```python
from build123d import *

# Parameters (mm, degrees)
SKETCH2_R          = 30
CUT_EXTRUDE1_DEPTH = 40


with BuildPart() as part:
    # Sketch1 → Revolve1 (revolve)
    with BuildSketch(Plane.XY, mode=Mode.PRIVATE) as revolve1_sk:
        Polygon((0, 0), (0, 10), (-20, 10), (-20, 20), (-40, 20), (-40, 30), (-60, 30), (-60, 40), (-80, 40), (-80, 50), (-100, 50), (-100, 60), (-120, 60), (-120, 70), (-140, 70), (-140, 40), (-180, 40), (-180, 0), align=None)
    revolve(revolve1_sk.sketch.rotate(Axis((0, 0, 0), (-1, 0, 0)), 90), axis=Axis((0, 0, 0), (-1, 0, 0)))  # turned: the seam where the file's is

    # Sketch2 → Cut-Extrude1 (cut)
    with BuildSketch(Plane.ZY.offset(180)):
        with Locations(Location((0, 0, 0), (0, 0, 180))):  # turned: the seam where the file's is
            Circle(SKETCH2_R)
    extrude(amount=-CUT_EXTRUDE1_DEPTH, mode=Mode.SUBTRACT)


solid = part.part
```
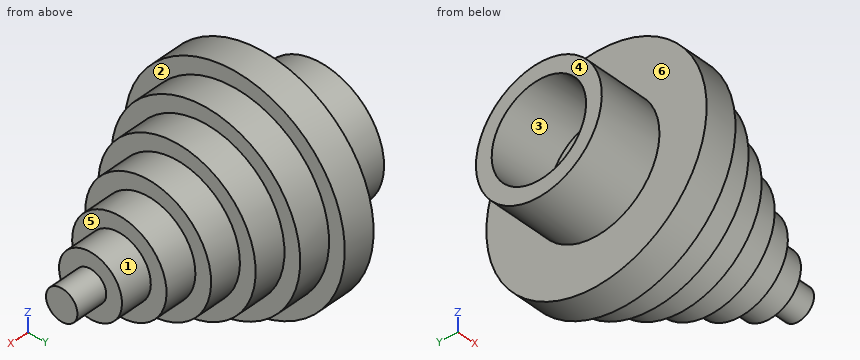
Verification items for the finished model (mm, model axes). Face numbers are marked on the shaded views. A direction names the side the tool comes from. Give positions to 0.01 mm unless a question says otherwise; leave off trailing zeros. Order: outer loops, then holes, each group sorted by start corner. A loop starts at its lowest first (then second) coordinate and runs counter-clockwise, first axis right, second up. Notation, with made-up numbers: M 16.5,36 L 36.5,36 A18 ccw 36.5,50 Z; hole C 3.5,79 d2. An arc over 180 degrees is marked long. Answer in a Markdown table with one row per item. Add a question column.
Item 1: Scan lines: probe 1 along Y at (x, z) = (-149, 0); probe 2 along X at (y, z) = (49, 20); probe 3 along X at (y, z) = (20, -17). Record each from-to range of solid material in increasing order. Write a range as from..to.
Item 2: Section check B-B, the plane x = -112. Enter the section's corners in (y, z).
Item 3: Section check D-D, the plane x = -133.5. Enter the section's corners in (y, z), and give its area (3 significant figures).
Item 4: Tool access check on the marked faces 4, 5 and 6. Record the directions out of +Z, -Z, +X, -X, +Y, -Y that give a thin tool (end or side, any length) a straight path to the whole face; none if there is none.
Item 5: Gauge pin test, flat ends, axial feed: pin 1 (5 mm diameter, centred on x = -76.5, y = -4, fed in from -Z); pin 2 (10 mm diameter, centred on x = -104, y = -15.5, fed in from -Z); pin 3 (10 mm diameter, centred on y = -14, z = -54.5, fed in from -X). Record the tip position at first contact, or that the pin passes through.
Item 6: Mould release check, pull along Y, two halves, no side actions. Record for the marked faces 1, 2 and 3: released by +Y, released by -Y, zero draft, split by the parting line, or undercut.
Item 7: Section check A-A, the plane z = -53. Enter the section's corners in (x, y), and give its area (3 significant figures).
Filled sheet:
| question | item | result |
|---|---|---|
| 1 | probe 1 | y = -40..-30, 30..40 |
| 1 | probe 2 | x = -140..-100 |
| 1 | probe 3 | x = -140..-40 |
| 2 | outline | C 0,0 d120 |
| 3 | outline | C 0,0 d140 |
| 3 | area | 15,400 mm^2 |
| 4 | face 4 | +Z, -Z, -X, +Y, -Y |
| 4 | face 5 | +X |
| 4 | face 6 | -X |
| 5 | pin 1 | stops at z = -39.97 |
| 5 | pin 2 | stops at z = -59.07 |
| 5 | pin 3 | stops at x = -140 |
| 6 | face 1 | split by the parting line |
| 6 | face 2 | zero draft |
| 6 | face 3 | undercut |
| 7 | outline | M -140,-45.73 L -120,-45.73 L -120,-28.12 L -100,-28.12 L -100,28.12 L -120,28.12 L -120,45.73 L -140,45.73 Z |
| 7 | area | 2,950 mm^2 |
